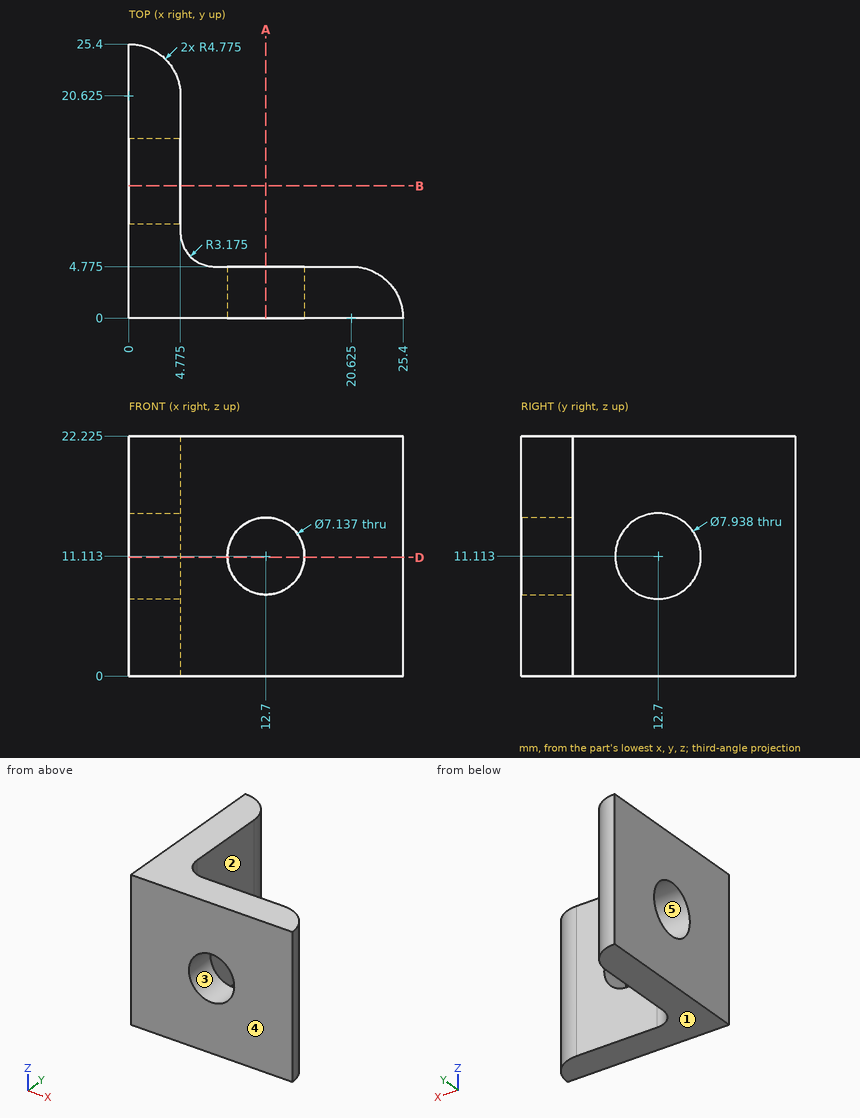
The drawing under review shows one solid part. Ordinate dimensions are in mm from its lowest x, y, z. A direction names the side the tool comes from. Round coordinates to 2 decimals unless told otherwise and drop trailing zeros. Loops run counter-clockwise (first coordinate to the right, second up) from the corner with the lowest first, then second, coordinate; pieces in that order, holes last. Notation, with made-up numbers: (19, -37.5) - (40, -37.5) arc R21 cw to (40, -20.5) - close; hole circle Ø6 at (23, 37.25). An arc over 180 degrees is marked (long way). Put each result on its own line as item: value. Start each with the question number.
1. Consider section B-B on y = 12.25. State the section outline as (x, z) points (1 decimal).
2. Consider section D-D on z = 11. State how many separate pieces and enclosed holes the cut face has, plus the area to 3 significant figures.
3. Mouldability with a two-part tool opening along Y and no side actions: class the marked faces 3, 4 and 5 as +Y half, -Y half, draft (parallel to the pull), parting line (faces both ways), or undercut.
4. Consider section A-A on x = 12.7. State the section outline as (y, z) points (1 decimal).
5. Insertion check: P1, Ø6.5, axis at y = 12, z = 10, coming from the +X side (1 decimal). The pin has a flat end and moves straight along its axis. Give the tip position at first contact, or say it passes through.
6. For probe 1 along Z at (x, y) = (12.7, 3.45) (1 decimal); probe 2 along X at (y, z) = (17.25, 19.75) (1 decimal), list the stretches that pass through material, from the lowest coordinate up. Write a range as [from, to].
7. For the marked faces 1 and 2, list the 3-axis set-ups (+Z, -Z, +X, -X, +Y, -Y) from which the entire face can be reached by the end or side of a thin tool; tool diameter is ignored.
Result sheet:
1. outline: (0, 0) - (4.8, 0) - (4.8, 7.2) - (0, 7.2) - close; (0, 15.1) - (4.8, 15.1) - (4.8, 22.2) - (0, 22.2) - close
2. separate pieces: 3
2. enclosed holes: 0
2. area: 140 mm^2
3. face 3: draft
3. face 4: -Y half
3. face 5: undercut
4. outline: (0, 0) - (4.8, 0) - (4.8, 7.5) - (0, 7.5) - close; (0, 14.7) - (4.8, 14.7) - (4.8, 22.2) - (0, 22.2) - close
5. P1: x = 4.8
6. probe 1: [0, 7.5], [14.7, 22.2]
6. probe 2: [0, 4.8]
7. face 1: -Z, +X, -X, +Y, -Y
7. face 2: +Z, -Z, +X, +Y
